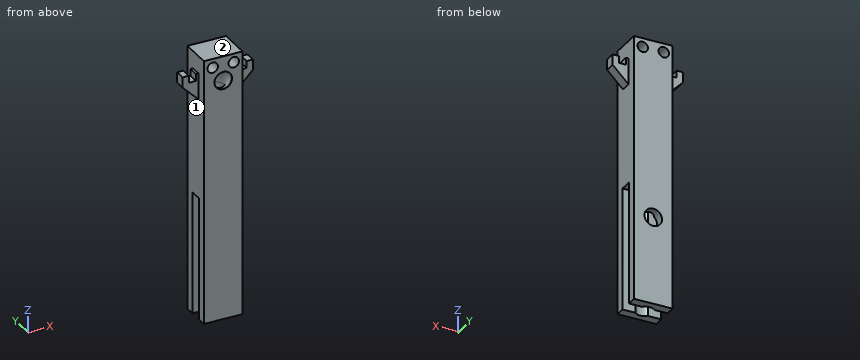
from build123d import *

# Parameters (mm, degrees)
SKETCH1_W           = 11
SKETCH1_H           = 76
BOSS_EXTRUDE1_DEPTH = 9
SKETCH4_R           = 2.5
SKETCH5_W           = 3
SKETCH5_H           = 3
BOSS_EXTRUDE2_DEPTH = 4.5
SKETCH6_W           = 2
SKETCH6_H           = 3
CUT_EXTRUDE2_DEPTH  = 2
BOSS_EXTRUDE3_DEPTH = 3
SKETCH10_W          = 11
SKETCH10_H          = 3.5
CUT_EXTRUDE5_DEPTH  = 35
CUT_EXTRUDE6_REACH  = 42.311
SKETCH11_R          = 2.5
CUT_EXTRUDE8_REACH  = 42.311
SKETCH8_R           = 1.5


with BuildPart() as part:
    # Sketch1 → Boss-Extrude1 (new body)
    with BuildSketch(Plane(origin=(0, 0, 0), x_dir=(1, 0, 0), z_dir=(0, 1, 0))):
        Rectangle(SKETCH1_W, SKETCH1_H)
    extrude(amount=BOSS_EXTRUDE1_DEPTH)

    # Cut-Sweep2: sweep along a path in Sketch3
    with BuildLine(Plane.ZY) as cut_sweep2_path:
        Line((-38, 4.5), (27, 4.5))
        ThreePointArc((27, 4.5), (29.828427125, 3.328427125), (31, 0.5))
        Line((31, 0.5), (31, 0))
    # Sketch4 → Cut-Sweep2 (sweep, cut)
    with BuildSketch(Plane(origin=(0, 0, -38), x_dir=(-1, 0, 0), z_dir=(0, 0, -1))):
        with Locations((0, 4.5)):
            Circle(SKETCH4_R)
    sweep(path=cut_sweep2_path.line, mode=Mode.SUBTRACT)

    # Sketch5 → Boss-Extrude2 (add)
    with BuildSketch(Plane.ZY.offset(5.5)):
        with Locations((31.5, 4.5)):
            Rectangle(SKETCH5_W, SKETCH5_H)
    boss_extrude2 = extrude(amount=BOSS_EXTRUDE2_DEPTH)

    # Mirror1: Boss-Extrude2 across plane
    add(boss_extrude2.mirror(Plane.ZY))

    # Sketch6 → Cut-Extrude2 (cut)
    with BuildSketch(Plane.XY.offset(33)):
        with Locations((-7.25, 4.5)):
            Rectangle(SKETCH6_W, SKETCH6_H)
    cut_extrude2 = extrude(amount=-CUT_EXTRUDE2_DEPTH, mode=Mode.SUBTRACT)

    # Mirror2: Cut-Extrude2 across plane
    add(cut_extrude2.mirror(Plane.ZY), mode=Mode.SUBTRACT)

    # Sketch7 → Boss-Extrude3 (add)
    with BuildSketch(Plane(origin=(0, 6, 0), x_dir=(1, 0, 0), z_dir=(0, 1, 0))):
        Polygon((-10, -30), (-5.5, -25.5), (-5.5, -30), align=None)
    boss_extrude3 = extrude(amount=-BOSS_EXTRUDE3_DEPTH)

    # Mirror3: Boss-Extrude3 across plane
    add(boss_extrude3.mirror(Plane.ZY))

    # Sketch10 → Cut-Extrude5 (cut)
    with BuildSketch(Plane(origin=(0, 0, -38), x_dir=(-1, 0, 0), z_dir=(0, 0, -1))):
        with Locations((0, 4.5)):
            Rectangle(SKETCH10_W, SKETCH10_H)
    extrude(amount=-CUT_EXTRUDE5_DEPTH, mode=Mode.SUBTRACT)

    # Sketch11 → Cut-Extrude6 (cut, up to next)
    with BuildSketch(Plane(origin=(0, 9, 0), x_dir=(1, 0, 0), z_dir=(0, 1, 0)), mode=Mode.PRIVATE) as cut_extrude6_sk1:
        with Locations(Location((0, 13, 0), (0, 0, 270))):
            Circle(SKETCH11_R)
    cut_extrude6_tool1 = extrude(cut_extrude6_sk1.sketch, amount=-CUT_EXTRUDE6_REACH, mode=Mode.PRIVATE) & part.part
    add(cut_extrude6_tool1.solids().sort_by_distance((0, 9, -13))[0], mode=Mode.SUBTRACT)

    # Sketch8 → Cut-Extrude8 (cut, up to next)
    with BuildSketch(Plane.XZ, mode=Mode.PRIVATE) as cut_extrude8_sk1:
        with Locations(Location((-3, 35.5, 0), (0, 0, 270))):
            Circle(SKETCH8_R)
    cut_extrude8_tool1 = extrude(cut_extrude8_sk1.sketch, amount=-CUT_EXTRUDE8_REACH, mode=Mode.PRIVATE) & part.part
    # Sketch8 → Cut-Extrude8 (cut, up to next)
    with BuildSketch(Plane.XZ, mode=Mode.PRIVATE) as cut_extrude8_sk2:
        with Locations(Location((3, 35.5, 0), (0, 0, 90))):
            Circle(SKETCH8_R)
    cut_extrude8_tool2 = extrude(cut_extrude8_sk2.sketch, amount=-CUT_EXTRUDE8_REACH, mode=Mode.PRIVATE) & part.part
    add(cut_extrude8_tool1.solids().sort_by_distance((-3, 0, 35.5))[0], mode=Mode.SUBTRACT)
    add(cut_extrude8_tool2.solids().sort_by_distance((3, 0, 35.5))[0], mode=Mode.SUBTRACT)


solid = part.part
Model file for the job. Use its own axes, mm. Face numbers are marked on the shaded views. Give positions to 0.01 mm unless a question says otherwise; leave off trailing zeros. Order: outer loops, then holes, each group sorted by start corner. A loop starts at its lowest first (then second) coordinate and runs counter-clockwise, first axis right, second up. Notation, with made-up numbers: (27, 83.5) - (83, 83.5) arc R15 cw to (83, 101.5) - close; hole circle Ø9 at (3, 38). An arc over 180 degrees is marked (long way). Write item = value, one per line. Start each with the question number.
1. Cut at B-B, the plane x = 0. List the corners of the cut face in (y, z), and give its area (3 significant figures).
2. Probe line 1 along X through (y, z) = (4.5, 35.5); line 2 along X through (y, z) = (6.9, -13); line 3 along X through (y, z) = (7.75, -33.5). List the from-to ranges inside material, lowest first.
3. Cut at C-C, the plane z = -13. List the corners of the cut face in (x, y), and give its area (3 significant figures).
4. Drop flat-ended pins along their axis: P1, Ø1.8, axis at x = 3, z = 35.5, coming from the +Y side; P2, Ø1.6, axis at x = 7.5, y = 5, coming from the +Z side; P3, Ø3.5, axis at x = -7.5, z = 30.5, coming from the -Y side; P4, Ø2.5, axis at y = 4, z = 6, coming from the -X side. Give the stop position or say it passes through.
5. Cut at D-D, the plane y = 7.75. List the corners of the cut face in (x, z), and give its area (3 significant figures).
6. Two-plate mould, pull along Z, no slides. Class the marked faces 1 and 2: pulls with the +Z half, pulls with the -Z half, needs draft (parallel to the pull), parting line crosses it, or undercut.
7. Cut at A-A, the plane z = -27. List the corners of the cut face in (x, y).
Taken from the geometry:
q1.outline = (0, -38) - (2, -38) - (2, 27) arc R1.5 ccw to (0.5, 28.5) - (0, 28.5) - close; (0, 33.5) - (0.5, 33.5) arc R6.5 cw to (7, 27) - (7, -10.5) - (9, -10.5) - (9, 38) - (0, 38) - close; (7, -38) - (9, -38) - (9, -15.5) - (7, -15.5) - close
q1.area = 315 mm²
q2.line_1 = -5.5 to -4.5, -1.5 to 1.5, 4.5 to 5.5
q2.line_2 = -5.5 to -2.5, 2.5 to 5.5
q2.line_3 = -5.5 to 5.5
q3.outline = (-5.5, 0) - (5.5, 0) - (5.5, 2.75) - (1.79, 2.75) arc R2.5 cw to (-1.79, 2.75) - (-5.5, 2.75) - close; (-5.5, 6.25) - (-2.5, 6.25) - (-2.5, 9) - (-5.5, 9) - close; (2.5, 6.25) - (5.5, 6.25) - (5.5, 9) - (2.5, 9) - close
q3.area = 44.9 mm²
q4.P1 = through
q4.P2 = 33
q4.P3 = 3
q4.P4 = -5.5
q5.outline = (-5.5, -38) - (5.5, -38) - (5.5, 38) - (-5.5, 38) - close; hole circle Ø3 at (-3, 35.5); hole circle Ø5 at (0, -13); hole circle Ø3 at (3, 35.5)
q5.area = 802 mm²
q6.face_1 = needs draft
q6.face_2 = pulls with the +Z half
q7.outline = (-5.5, 0) - (5.5, 0) - (5.5, 2.75) - (1.79, 2.75) arc R2.5 cw to (-1.79, 2.75) - (-5.5, 2.75) - close; (-5.5, 6.25) - (-1.79, 6.25) arc R2.5 cw to (1.79, 6.25) - (5.5, 6.25) - (5.5, 9) - (-5.5, 9) - close
